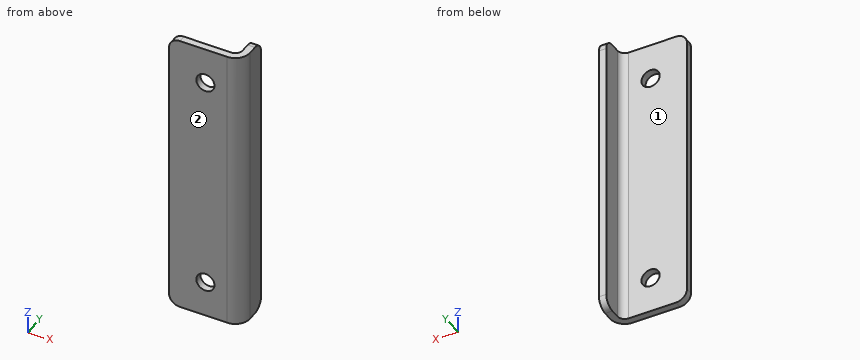
from build123d import *

# Parameters (mm, degrees)
SKETCH1_W                    = 20
SKETCH1_H                    = 80
BASE_FLANGE1_DEPTH           = 2
EDGE_FLANGE1_STRIP_W         = 12
EDGE_FLANGE1_STRIP_H         = 2
EDGE_FLANGE1_STRIP_CUT_DEPTH = 80
EDGE_FLANGE1_DEPTH           = 80
F_5_0MM_DOWEL_HOLE1_D        = 5
FILLET1_R                    = 3


# Sheet-metal steps are written as plain solids
with BuildPart() as part:
    # Sketch1 → Base-Flange1 (new body)
    with BuildSketch(Plane(origin=(0, 0, 0), x_dir=(1, 0, 0), z_dir=(0, 1, 0))):
        Rectangle(SKETCH1_W, SKETCH1_H)
    extrude(amount=BASE_FLANGE1_DEPTH)

    # Edge-Flange1 strip (across the edge) → Edge-Flange1 strip cut (cut)
    with BuildSketch(Plane(origin=(10, 2, 40), x_dir=(-1, 0, 0), z_dir=(0, 0, -1))):
        with Locations((-2, -1)):
            Rectangle(EDGE_FLANGE1_STRIP_W, EDGE_FLANGE1_STRIP_H)
    extrude(amount=EDGE_FLANGE1_STRIP_CUT_DEPTH, mode=Mode.SUBTRACT)

    # Edge-Flange1 section (across the edge) → Edge-Flange1 (add)
    with BuildSketch(Plane(origin=(10, 2, 40), x_dir=(-1, 0, 0), z_dir=(0, 0, -1))):
        with BuildLine():
            Line((0, 2), (0, 7.5))
            Line((0, 7.5), (2, 7.5))
            Line((2, 7.5), (2, 2))
            ThreePointArc((2, 2), (2.585786438, 0.585786438), (4, 0))
            Line((4, 0), (4, -2))
            ThreePointArc((4, -2), (1.171572875, -0.828427125), (0, 2))
        make_face()
    extrude(amount=EDGE_FLANGE1_DEPTH)

    # Ø5.0mm Dowel Hole1 (through all)
    with Locations(Plane(origin=(0, 2, 0), x_dir=(1, 0, 0), z_dir=(0, 1, 0))):
        with Locations((0, 30), (0, -30)):
            Hole(F_5_0MM_DOWEL_HOLE1_D / 2)

    # Fillet1
    fillet1_edges = [part.edges().sort_by_distance(p)[0] for p in [
        (9, 9.5, 40),
        (9, 9.5, -40),
        (-10, 1, -40),
        (-10, 1, 40),
    ]]
    fillet(fillet1_edges, radius=FILLET1_R)


solid = part.part
Work out the finished part from the listing and answer in its coordinate system (mm). Face numbers are marked on the shaded views. A direction names the side the tool comes from. Round coordinates to 2 decimals unless told otherwise and drop trailing zeros. Loops run counter-clockwise (first coordinate to the right, second up) from the corner with the lowest first, then second, coordinate; pieces in that order, holes last. Notation, with made-up numbers: (-20.5, 12) -> (3.5, 12) arc R6 cw to (3.5, 21) -> close; hole circle Ø8 at (12, -1.5). An arc over 180 degrees is marked (long way). Use one line per item in the form item = value.
(1) Flat-ended cylindrical pins translate along their axes: P1, Ø3, axis at x = 0, z = -30, coming from the -Y side (3 decimals); P2, Ø6, axis at x = 0, z = 30, coming from the -Y side; P3, Ø8, axis at x = -6, z = -1, coming from the +Y side; P4, Ø3, axis at y = 5.5, z = -10.5, coming from the -X side. Find the tip coordinate at first contact, or state that the pin passes through.
Answer list:
P1 = through
P2 = 0
P3 = 2
P4 = 8
(2) A tool of negligible diameter and unlimited length cuts with its end or side. For the marked faces 1 and 2, from which of +Z, -Z, +X, -X, +Y, -Y can it reach the whole face along a straight path? Write none if from no direction.
Answer list:
face_1 = +Z, -Z, -X, +Y
face_2 = +Z, -Z, +X, -X, -Y
(3) Find section D-D on x = -3.5. Give the vertices of the cut face in (y, z).
Answer list:
outline = (0, -40) -> (2, -40) -> (2, 40) -> (0, 40) -> close
(4) Straight lines are drawn through the part: line 1 (Z direction, x = 0, y = 1.05); line 2 (Y direction, x = -5.75, z = -14); line 3 (X direction, y = 9.25, z = -23). For each, find the intervals that lie inside material, in ascending order.
Answer list:
line_1 = -40 to -32.5, -27.5 to 27.5, 32.5 to 40
line_2 = 0 to 2
line_3 = 8 to 10
(5) Find section C-C on y = 8.5. Give the vertices of the cut face in (x, z), then the cut area to 3 significant figures.
Answer list:
outline = (8, -39.24) -> (10, -39.24) -> (10, 39.24) -> (8, 39.24) -> close
area = 157 mm2
(6) Find section B-B on z = 30. Give the vertices of the cut face in (x, y).
Answer list:
outline = (-10, 0) -> (-2.5, 0) -> (-2.5, 2) -> (-10, 2) -> close; (2.5, 0) -> (6, 0) arc R4 ccw to (10, 4) -> (10, 9.5) -> (8, 9.5) -> (8, 4) arc R2 cw to (6, 2) -> (2.5, 2) -> close
(7) Find section A-A on x = 0. Give the vertices of the cut face in (y, z).
Answer list:
outline = (0, -40) -> (2, -40) -> (2, -32.5) -> (0, -32.5) -> close; (0, -27.5) -> (2, -27.5) -> (2, 27.5) -> (0, 27.5) -> close; (0, 32.5) -> (2, 32.5) -> (2, 40) -> (0, 40) -> close
